from build123d import *

# Parameters (mm, degrees)
SKETCH1_W           = 71.7
SKETCH1_H           = 48
BOSS_EXTRUDE1_DEPTH = 1
SKETCH2_R           = 1.4
CUT_EXTRUDE1_DEPTH  = 44.153476106
BOSS_EXTRUDE2_START = -1
SKETCH3_W           = 62
SKETCH3_H           = 39.8
BOSS_EXTRUDE2_DEPTH = 4
SKETCH4_W           = 55.01
SKETCH4_H           = 27.49
CUT_EXTRUDE2_DEPTH  = 0.5
SKETCH5_R           = 0.45
CUT_EXTRUDE3_DEPTH  = 44.246069186
LPATTERN1_COUNT     = 4
LPATTERN1_PITCH     = 2.54
SKETCH6_R           = 0.45
CUT_EXTRUDE4_DEPTH  = 44.246069186
LPATTERN2_COUNT     = 4
LPATTERN2_PITCH     = 2.54
SKETCH7_W           = 15
SKETCH7_H           = 15
BOSS_EXTRUDE3_DEPTH = 0.1


with BuildPart() as part:
    # Sketch1 → Boss-Extrude1 (new body)
    with BuildSketch(Plane(origin=(0, 0, 0), x_dir=(1, 0, 0), z_dir=(0, 1, 0))):
        Rectangle(SKETCH1_W, SKETCH1_H)
    extrude(amount=BOSS_EXTRUDE1_DEPTH)

    # Sketch2 → Cut-Extrude1 (cut, through all)
    with BuildSketch(Plane(origin=(0, 1, 0), x_dir=(1, 0, 0), z_dir=(0, 1, 0))):
        with Locations(Location((-32.8, 21.575, 0), (0, 0, 270))):
            Circle(SKETCH2_R)
        with Locations(Location((32.8, 21.575, 0), (0, 0, 270))):
            Circle(SKETCH2_R)
        with Locations(Location((-32.8, -21.575, 0), (0, 0, 270))):
            Circle(SKETCH2_R)
        with Locations(Location((32.8, -21.575, 0), (0, 0, 270))):
            Circle(SKETCH2_R)
    extrude(amount=-CUT_EXTRUDE1_DEPTH, mode=Mode.SUBTRACT)

    # Sketch3 → Boss-Extrude2 (add)
    with BuildSketch(Plane(origin=(0, 1, 0), x_dir=(1, 0, 0), z_dir=(0, 1, 0)).offset(BOSS_EXTRUDE2_START)):
        Rectangle(SKETCH3_W, SKETCH3_H)
    extrude(amount=BOSS_EXTRUDE2_DEPTH)

    # Sketch4 → Cut-Extrude2 (cut)
    with BuildSketch(Plane(origin=(0, 4, 0), x_dir=(1, 0, 0), z_dir=(0, 1, 0))):
        with Locations((0, 2.976)):
            Rectangle(SKETCH4_W, SKETCH4_H)
    extrude(amount=-CUT_EXTRUDE2_DEPTH, mode=Mode.SUBTRACT)

    # Sketch5 → Cut-Extrude3 (cut, through all)
    with BuildSketch(Plane(origin=(0, 1, 0), x_dir=(1, 0, 0), z_dir=(0, 1, 0))):
        with Locations(Location((-4.66, 21.55, 0), (0, 0, 270))):
            Circle(SKETCH5_R)
    cut_extrude3 = extrude(amount=-CUT_EXTRUDE3_DEPTH, mode=Mode.SUBTRACT)

    # LPattern1: Cut-Extrude3 ×4
    with Locations(*[(i * LPATTERN1_PITCH, 0, 0) for i in range(1, LPATTERN1_COUNT)]):
        add(cut_extrude3, mode=Mode.SUBTRACT)

    # Sketch6 → Cut-Extrude4 (cut, through all)
    with BuildSketch(Plane(origin=(0, 1, 0), x_dir=(1, 0, 0), z_dir=(0, 1, 0))):
        with Locations(Location((-34.05, 4.11, 0), (0, 0, 270))):
            Circle(SKETCH6_R)
    cut_extrude4 = extrude(amount=-CUT_EXTRUDE4_DEPTH, mode=Mode.SUBTRACT)

    # LPattern2: Cut-Extrude4 ×4
    with Locations(*[(0, 0, i * LPATTERN2_PITCH) for i in range(1, LPATTERN2_COUNT)]):
        add(cut_extrude4, mode=Mode.SUBTRACT)

    # Sketch7 → Boss-Extrude3 (add)
    with BuildSketch(Plane(origin=(0, 3.5, 0), x_dir=(1, 0, 0), z_dir=(0, 1, 0))):
        with Locations((-13.7525, 2.976)):
            Rectangle(SKETCH7_W, SKETCH7_H)
    boss_extrude3 = extrude(amount=BOSS_EXTRUDE3_DEPTH)

    # Mirror1: Boss-Extrude3 across plane
    add(boss_extrude3.mirror(Plane(origin=(0, 0, 0), x_dir=(0, 0, 1), z_dir=(1, 0, 0))))


solid = part.part
The listing builds one solid part. Answer for the finished solid, in the listing's coordinates (mm). A direction names the side the tool comes from. Give positions to 0.01 mm unless a question says otherwise; leave off trailing zeros. Order: outer loops, then holes, each group sorted by start corner. A loop starts at its lowest first (then second) coordinate and runs counter-clockwise, first axis right, second up. Notation, with made-up numbers: (10.5, 8) - (17.5, 8) arc R12 cw to (17.5, 20) - close; hole circle Ø4 at (0, 78). An arc over 180 degrees is marked (long way). One line per item, written item: value. Start each with the question number.
1) A cutting plane is placed at A-A on x = 20. Give the vertices of the cut face in (y, z).
2) A cutting plane is placed at B-B on y = 2. Give the vertices of the cut face in (x, z).
3) Find the intervals of material crossed by L1, parallel to Z at x = 27, y = 3.65; L2, parallel to X at y = 0.2, z = -1.57; L3, parallel to X at y = 3.65, z = -14 (3 decimals), in increasing order.
4) A tool of negligible diameter and unlimited length cuts with its end or side. For faces 4 (the face through (0, 2, -19.9)), 5 (the face through (-14, 3.6, -3)), 6 (the face through (31.948, 0.507, -22.686)), 7 (the face through (-31, 2, 0)), from which of +Z, -Z, +X, -X, +Y, -Y can it reach the whole face along a straight path? Write none if from no direction.
5) Given pin 1 Ø8 at (x, z) = (-3.5, 9) entering from +Y; pin 2 Ø12 at (x, z) = (-13.5, -5.5) entering from +Y; pin 3 Ø0.9 at (x, y) = (-13, 2) entering from +Z; pin 4 Ø1.5 at (y, z) = (2, -3.5) entering from -X, each flat-ended and moving along its own axis, determine where each tip first touches the part or whether it passes through.
6) The mould has two halves that part along X. Classify faces 1 (the face through (31.948, 0.507, 20.464)), 2 (the face through (0, 2, 19.9)), 3 (the face through (31, 2, 0)): released by +X, released by -X, zero draft, split by the parting line, or undercut.
Answer sheet:
1. outline: (0, -24) - (1, -24) - (1, -19.9) - (4, -19.9) - (4, -16.72) - (3.5, -16.72) - (3.5, -10.48) - (3.6, -10.48) - (3.6, 4.52) - (3.5, 4.52) - (3.5, 10.77) - (4, 10.77) - (4, 19.9) - (1, 19.9) - (1, 24) - (0, 24) - close
2. outline: (-31, -19.9) - (31, -19.9) - (31, 19.9) - (-31, 19.9) - close
3. L1: z = -19.9 to -16.72, 10.77 to 19.9
3. L2: x = -35.85 to -34.5, -33.6 to 35.85
3. L3: x = -31 to -27.505, 27.505 to 31
4. face 4: -Z, +X, -X, +Y
4. face 5: +Y
4. face 6: +Y, -Y
4. face 7: +Z, -Z, -X, +Y
5. pin 1: stops at y = 4
5. pin 2: stops at y = 3.6
5. pin 3: stops at z = 19.9
5. pin 4: stops at x = -31
6. face 1: undercut
6. face 2: zero draft
6. face 3: released by +X
